Here's how the part is built. I have some questions about the finished solid (model axes, mm). Face numbers are marked on the shaded views. A direction names the side the tool comes from. Coordinates: 2 decimals unless noted, no trailing zeros. Loops run counter-clockwise (first coordinate to the right, second up) from the corner with the lowest first, then second, coordinate; pieces in that order, holes last. Notation, with made-up numbers: M 31,8.5 L 36,8.5 A33 cw 36,45.5 Z; hole C 55.5,-34 d6. An arc over 180 degrees is marked long. Use one line per item in the form item = value. Start each with the question number.
(1) Thinking about a two-plate mould opening in X: for the marked faces 6, 7, 8 and 9, which applies, +X half, -X half, draft (parallel to the pull), parting line (faces both ways), or undercut?
(2) Please list where these lines run through material, in increasing order: L1, parallel to Y at x = 28.5, z = -4; L2, parallel to Y at x = -1, z = 6.5; L3, parallel to X at y = -11, z = -22.
(3) On a 3-axis mill with a long thin cutter (end or side, diameter ignored), from which of +Z, -Z, +X, -X, +Y, -Y can I reach the whole of each face in a straight line? I mean the marked faces 1, 2, 3, 4 and 5. Say none if no direction works.
(4) Will these pins go through, and if not, where does the flat tip stop? P1, Ø13.5, axis at x = 11, z = -20, coming from the -Y side; P2, Ø2, axis at x = 44.5, y = -12.5, coming from the -Z side; P3, Ø8, axis at x = 12, z = -44.5, coming from the +Y side.
(5) Imagine slicing it at B-B, the plane y = 21.5. Please give me the cut outline in (x, z).
(6) Imagine slicing it at C-C, the plane z = -32. State how many separate pieces and enclosed holes the cut face has, and give its area (3 significant figures).
(7) Imagine slicing it at A-A, the plane y = 0. Please give me the cut outline in (x, z), and give its area (3 significant figures).
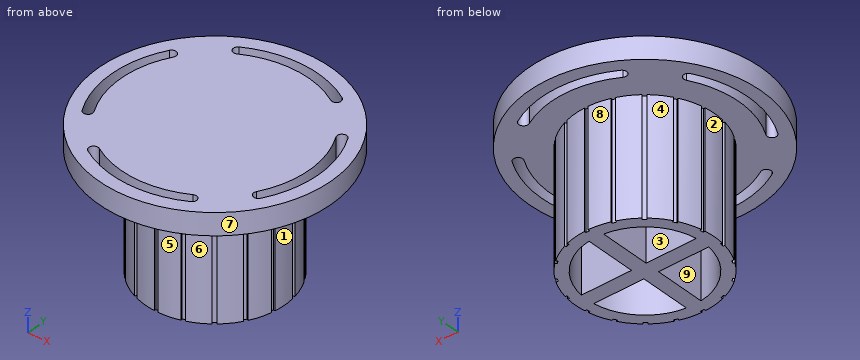
Autodesk Inventor part; units mm, degrees
ref_plane "YZ Plane" through (0, 0, 0) normal (1, 0, 0) x (0, 1, 0)
ref_plane "XZ Plane" through (0, 0, 0) normal (0, 1, 0) x (-1, 0, 0)
ref_plane "XY Plane" through (0, 0, 0) normal (0, 0, 1) x (1, 0, 0)
sketch "Sketch1" plane through (0, 0, 0) normal (0, 0, 1) x (1, 0, 0)
  circle A0 centre (0, 0) radius 38.1
  circle A1 centre (0, 0) radius 63.5
  circle A2 centre (0, 0) radius 31.75
  dimension "d1" = 76.2
  dimension "d7" = 6.35
  dimension "d45" = 127
extrude "Extrusion2" add sketch "Sketch1" along normal blind 12 contours A0 | A1 | A2
extrude "Extrusion3" add sketch "Sketch1" against normal blind 63.5 contours A0
sketch "Sketch6" plane through (0, 0, 12) normal (0, 0, 1) x (1, 0, 0)
  arc A0 (26.9875, 46.7437) -> (-26.9875, 46.7437) centre (0, 0) ccw construction
  arc A1 (28.2638, 48.9544) -> (-28.2639, 48.9544) centre (0, 0) ccw
  arc A2 (25.7111, 44.533) -> (-25.7112, 44.533) centre (0, 0) ccw
  arc A3 (25.7111, 44.533) -> (28.2638, 48.9544) centre (26.9875, 46.7437) ccw
  arc A4 (-28.2639, 48.9544) -> (-25.7112, 44.533) centre (-26.9875, 46.7437) ccw
  line L0 (0, 0) -> (26.9875, 46.7437) construction
  line L1 (0, 0) -> (53.975, 0) construction
  line L2 (0, 0) -> (-26.9875, 46.7437) construction
  dimension "d26" = 53.975
  dimension "d27" = 60
  dimension "d28" = 60
  dimension "d29" = 5.1054
extrude "Extrusion7" cut sketch "Sketch6" against normal through all
pattern_circular "Circular Pattern1" count 4 over 360 about axis through (0, 0, -10) along (0, 0, 1) of "Extrusion7"
sketch "Sketch8" plane through (0, 0, -63.5) normal (0, 0, -1) x (-1, 0, 0)
  circle A0 centre (0, 0) radius 38.1
  arc A1 (0, 38.1) -> (-1.016, 38.0865) centre (0, 0) ccw
  line L0 (0, 0) -> (0, 38.1) construction
  line L1 (0, 38.1) -> (0, 37.084)
  line L2 (0, 37.084) -> (-1.016, 37.084)
  line L3 (-1.016, 37.084) -> (-1.016, 38.0865)
  circle A2 centre (0, 0) radius 38.1
  circle A3 centre (0, 0) radius 38.1
  line L4 (0, 37.084) -> (1.016, 37.084)
  line L5 (1.016, 37.084) -> (1.016, 38.0865)
  dimension "d35" = 1.016
  dimension "d36" = 1.016
extrude "Extrusion9" cut sketch "Sketch8" against normal up to surface (63.5 mm away) contours L5 L4 L1 A0 | A0 L1 L2 L3
sketch "Sketch3" plane through (0, 0, 12) normal (0, 0, 1) x (1, 0, 0)
  ellipse E0 centre (0, 0) end of major axis (57.15, 0) minor radius 60.8178
  circle A0 centre (0, 0) radius 63.5
  circle A1 centre (0, 0) radius 63.5
  point P0 (-57.15, 0)
  point P1 (57.15, 0)
  dimension "d11" = 60.8178
  dimension "d12" = 57.15
pattern_circular "Circular Pattern2" count 18 over 360 about axis through (0, 0, -10) along (0, 0, 1) of "Extrusion9"
sketch "Sketch9" plane through (0, 0, 0) normal (0, 0, -1) x (-1, 0, 0)
  point P0 (0, 0)
sketch "Sketch10" plane through (0, 0, 0) normal (0, 0, -1) x (-1, 0, 0)
  circle A0 centre (0, 0) radius 31.75
  arc A1 (-31.497, 4) -> (-31.497, -4) centre (0, 0) ccw
  arc A2 (-4, -31.497) -> (4, -31.497) centre (0, 0) ccw
  arc A3 (31.497, -4) -> (31.497, 4) centre (0, 0) ccw
  arc A4 (4, 31.497) -> (-4, 31.497) centre (0, 0) ccw
  line L0 (-31.497, 4) -> (-4, 4)
  line L1 (4, 4) -> (31.497, 4)
  line L2 (-4, 31.497) -> (-4, 4)
  line L3 (-4, -4) -> (-4, -31.497)
  line L4 (4, 31.497) -> (4, 4)
  line L5 (4, -4) -> (4, -31.497)
  line L6 (-31.497, -4) -> (-4, -4)
  line L7 (4, -4) -> (31.497, -4)
extrude "Extrusion10" add sketch "Sketch10" along normal up to surface (63.5 mm away) contours A0 L7 L5 L3 L6 L0 L2 L4 L1
equation "\"d1\" = insideDiameterforPipe"
equation "\"d45\" = outsideDiameter"
equation "\"d8\" = insertDepthIntoPipe"
equation "\"d26\" = slotRadius"
equation "\"d28\" = totalAngleForSlot"
equation "\"d29\" = widthOfSlot"
equation "\"d11\" = 0.5 * elipseMajorDiameter"
equation "\"d12\" = 0.5 * elipseMinorDiameter"
equation "\"insideDiameterforPipe\" = 76.2"
equation "\"outsideDiameter\" = 127"
equation "\"elipseMajorDiameter\" = 121.63552"
equation "\"elipseMinorDiameter\" = 114.3"
equation "\"widthOfSlot\" = 5.1054"
equation "\"totalAngleForSlot\" = 60deg"
equation "\"slotDiameter\" = 0.5 * pipeExteriorDiameter + 0.5 * outsideDiameter"
equation "\"slotRadius\" = 0.5 * slotDiameter"
equation "\"pipeExteriorDiameter\" = 88.9"
equation "\"insertDepthIntoPipe\" = 63.5"
properties part number "3inPvcCap" material "PC/ABS Plastic"
Answer:
q1.face_6 = +X half
q1.face_7 = parting line
q1.face_8 = -X half
q1.face_9 = undercut
q2.L1 = -25.29 to -13.99, -4 to 4, 13.99 to 25.29
q2.L2 = -63.49 to -56.52, -51.41 to 51.41, 56.52 to 63.49
q2.L3 = -36.48 to -29.78, -4 to 4, 29.78 to 36.48
q3.face_1 = -Z, +X
q3.face_2 = -Z, -X
q3.face_3 = -Z
q3.face_4 = -Z, -X, +Y
q3.face_5 = -Z, +X, -Y
q4.P1 = -37.86
q4.P2 = 0
q4.P3 = 37.25
q5.outline = M -59.75,0 L -52.28,0 L -52.28,12 L -59.75,12 Z; M -46.71,0 L -31.45,0 L -31.45,-63.5 L -23.36,-63.5 L -23.36,0 L -4,0 L -4,-63.5 L 4,-63.5 L 4,0 L 23.36,0 L 23.36,-63.5 L 31.45,-63.5 L 31.45,0 L 46.71,0 L 46.71,12 L -46.71,12 Z; M 52.28,0 L 59.75,0 L 59.75,12 L 52.28,12 Z
q6.separate_pieces = 1
q6.enclosed_holes = 4
q6.area = 2,310 mm²
q7.outline = M -63.5,0 L -56.53,0 L -56.53,12 L -63.5,12 Z; M -51.42,0 L -38.1,0 L -38.1,-63.5 L 38.1,-63.5 L 38.1,0 L 51.42,0 L 51.42,12 L -51.42,12 Z; M 56.53,0 L 63.5,0 L 63.5,12 L 56.53,12 Z
q7.area = 6,240 mm²
